Geometry check sheet. Reference: the model listing, model coordinates, mm. Face numbers are marked on the shaded views. Round coordinates to 2 decimals unless told otherwise and drop trailing zeros. Write each loop counter-clockwise with the first axis right and the second up, starting at its lowest first coordinate (ties: lowest second). Pieces come first, ordered by that corner, then holes. Notation, with made-up numbers: (31, 36) - (79, 36) arc R30 cw to (79, 63) - close; hole circle Ø5 at (64, -5.5). An arc over 180 degrees is marked (long way). Return JSON: item names as keys, results as strings.
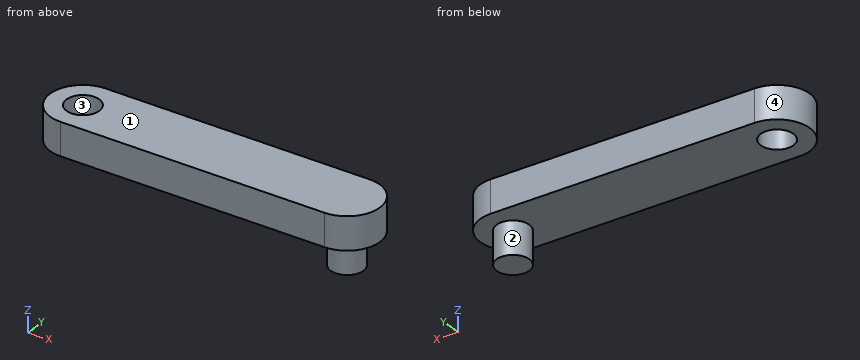
Autodesk Inventor part; units mm, degrees
ref_plane "YZ Plane" through (0, 0, 0) normal (1, 0, 0) x (0, 1, 0)
ref_plane "XZ Plane" through (0, 0, 0) normal (0, 1, 0) x (-1, 0, 0)
ref_plane "XY Plane" through (0, 0, 0) normal (0, 0, 1) x (1, 0, 0)
sketch "Sketch1" plane through (0, 0, 0) normal (0, 0, 1) x (1, 0, 0)
  line L0 (-17, 4) -> (23, 4) construction
  line L1 (-17, -1) -> (23, -1)
  line L2 (23, 9) -> (-17, 9)
  arc A0 (-17, 9) -> (-17, -1) centre (-17, 4) ccw
  arc A1 (23, -1) -> (23, 9) centre (23, 4) ccw
  circle A2 centre (-17, 4) radius 2.5
  circle A3 centre (23, 4) radius 2.5
  point P0 (0, 0)
  point P1 (3, 4)
  dimension "d0" = 40
  dimension "d1" = 10
  dimension "d2" = 5
extrude "Extrusion1" add sketch "Sketch1" along normal blind 5 contours A0 L2 A1 L1 | A3
extrude "Extrusion2" add sketch "Sketch1" against normal blind 5 contours A3
(1) Material ranges on line 1 along Y through (x, z) = (-17, 3); line 2 along Z through (x, y) = (12.5, 3.25); line 3 along X through (y, z) = (2, 4.25), recorded low to high. Write a range as [from, to].
Response values:
{"line 1": "y = [-1, 1.5], [6.5, 9]", "line 2": "z = [0, 5]", "line 3": "x = [-21.58, -18.5], [-15.5, 27.58]"}
(2) Section check D-D, the plane x = -5.5. Enter the section's corners in (y, z).
Response values:
{"outline": "(-1, 0) - (9, 0) - (9, 5) - (-1, 5) - close"}
(3) Section check C-C, the plane z = 1. Enter the section's corners in (x, y), plus the area to 3 significant figures.
Response values:
{"outline": "(-17, -1) - (23, -1) arc R5 ccw to (23, 9) - (-17, 9) arc R5 ccw to start; hole circle Ø5 at (-17, 4)", "area": "459 mm^2"}
(4) Section check B-B, the plane x = -16.5. Enter the section's corners in (y, z), plus the area to 3 significant figures.
Response values:
{"outline": "(-1, 0) - (1.55, 0) - (1.55, 5) - (-1, 5) - close; (6.45, 0) - (9, 0) - (9, 5) - (6.45, 5) - close", "area": "25.5 mm^2"}
(5) Gauge pin test, flat ends, axial feed: pin 1 (4 mm diameter, centred on x = -17, y = 4, fed in from -Z); pin 2 (6 mm diameter, centred on x = -1, z = -2, fed in from -Y); pin 3 (3 mm diameter, centred on x = 7, y = 4.5, fed in from -Z). Record the tip position at first contact, or that the pin passes through.
Response values:
{"pin 1": "passes through", "pin 2": "stops at y = -1", "pin 3": "stops at z = 0"}
(6) Release check for a two-part mould opening along X. For the marked faces 1, 2, 3 and 4 record: pulls with the +X half, pulls with the -X half, needs draft (parallel to the pull), parting line crosses it, or undercut.
Response values:
{"face 1": "needs draft", "face 2": "parting line crosses it", "face 3": "undercut", "face 4": "pulls with the -X half"}
(7) Section check A-A, the plane y = 4. Enter the section's corners in (x, z), plus the area to 3 significant figures.
Response values:
{"outline": "(-22, 0) - (-19.5, 0) - (-19.5, 5) - (-22, 5) - close; (-14.5, 0) - (20.5, 0) - (20.5, -5) - (25.5, -5) - (25.5, 0) - (28, 0) - (28, 5) - (-14.5, 5) - close", "area": "250 mm^2"}
